from build123d import *

# Parameters (mm, degrees)
SKETCH_1_W      = 3.5
SKETCH_1_H      = 2.1
SKETCH_1_W_2    = 3
SKETCH_1_H_2    = 1.6
EXTRUDE_1_DEPTH = 9.2
FILLET_1_R      = 0.25


with BuildPart() as part:
    # 草图1 → 凸台-拉伸1 (new body)
    with BuildSketch(Plane(origin=(0, 0, 0), x_dir=(0, 0, -1), z_dir=(1, 0, 0))):
        Rectangle(SKETCH_1_W, SKETCH_1_H)
        Rectangle(SKETCH_1_W_2, SKETCH_1_H_2, mode=Mode.SUBTRACT)
    extrude(amount=EXTRUDE_1_DEPTH)

    # 圆角1
    fillet_1_edges = [part.edges().sort_by_distance(p)[0] for p in [
        (4.6, -1.05, 1.75),
        (4.6, 1.05, 1.75),
        (4.6, 1.05, -1.75),
        (4.6, -1.05, -1.75),
    ]]
    fillet(fillet_1_edges, radius=FILLET_1_R)


solid = part.part
Source: CAD feature listing. Evaluate the final solid. Frame: model axes, mm. A direction names the side the tool comes from. Round coordinates to 2 decimals unless told otherwise and drop trailing zeros. Loops run counter-clockwise (first coordinate to the right, second up) from the corner with the lowest first, then second, coordinate; pieces in that order, holes last. Notation, with made-up numbers: (-17.5, 34) -> (-2.5, 34) arc R19 cw to (-2.5, 47) -> close; hole circle Ø6 at (6.5, 70). An arc over 180 degrees is marked (long way). Answer as a JSON object with one key per item and string values. Group by question number.
Q1. Section query B-B (z = -0.65). Output: boundary loops of the cut face in (x, y).
Q2. Ray query, line 1 (Z direction, x = 2.25, y = -0.6); line 2 (Y direction, x = 4.75, z = 0.65); line 3 (Z direction, x = 2.75, y = 0.9). Return the intervals inside material, ascending. Write a range as from..to.
Q3. Section query C-C (x = 6.25). Output: boundary loops of the cut face in (y, z), plus the area to 3 significant figures.
Q4. Access query for faces 4 (the flat face through (5, 0.8, 0)), 5 (the flat face through (5, 0, 1.75)). Directions: +Z, -Z, +X, -X, +Y, -Y. A direction counts if a zero-diameter tool reaches every point of the face in a straight line with its end or side. Return the directions, or none.
Q5. Mould query, pull axis Z, two halves, no side actions, for faces 1 (the flat face through (5, 0, -1.75)), 2 (the flat face through (5, -0.8, 0)), 3 (the flat face through (5, 1.05, 0)). Classes: pulls with the +Z half, pulls with the -Z half, needs draft (parallel to the pull), parting line crosses it, or undercut.
Q6. Section query A-A (y = 0.45). Output: boundary loops of the cut face in (x, z), plus the area to 3 significant figures.
Q7. Contact query for a flat-ended pin moving along its axis: P1, Ø1, axis at y = -0.5, z = 1, coming from the +X side. Output: stop coordinate, or through.
Completed:
{
 "1": {"outline": "(0, -1.05) -> (9.2, -1.05) -> (9.2, -0.8) -> (0, -0.8) -> close; (0, 0.8) -> (9.2, 0.8) -> (9.2, 1.05) -> (0, 1.05) -> close"},
 "2": {"line 1": "-1.75..-1.5, 1.5..1.75", "line 2": "-1.05..-0.8, 0.8..1.05", "line 3": "-1.73..1.73"},
 "3": {"outline": "(-1.05, -1.5) arc R0.25 ccw to (-0.8, -1.75) -> (0.8, -1.75) arc R0.25 ccw to (1.05, -1.5) -> (1.05, 1.5) arc R0.25 ccw to (0.8, 1.75) -> (-0.8, 1.75) arc R0.25 ccw to (-1.05, 1.5) -> close; hole (-0.8, -1.5) -> (0.8, -1.5) -> (0.8, 1.5) -> (-0.8, 1.5) -> close", "area": "2.50 mm²"},
 "4": {"face 4": "+X, -X", "face 5": "+Z, +X, -X, +Y, -Y"},
 "5": {"face 1": "pulls with the -Z half", "face 2": "undercut", "face 3": "needs draft"},
 "6": {"outline": "(0, -1.75) -> (9.2, -1.75) -> (9.2, -1.5) -> (0, -1.5) -> close; (0, 1.5) -> (9.2, 1.5) -> (9.2, 1.75) -> (0, 1.75) -> close", "area": "4.60 mm²"},
 "7": {"P1": "x = 9.2"}
}
